from build123d import *

# Parameters (mm, degrees)
BOSS_EXTRUDE3_DEPTH = 3
FILLET1_R           = 2
SKETCH12_R          = 2.1
CUT_EXTRUDE5_DEPTH  = 10
FILLET5_R           = 4
FILLET6_R           = 3
FILLET7_R           = 10
CUT_EXTRUDE9_DEPTH  = 1.5
SKETCH17_W          = 7.951649766
SKETCH17_H          = 5.272619773
SKETCH17_W_2        = 3.894064167
SKETCH17_H_2        = 6.195846789
CUT_EXTRUDE10_DEPTH = 1.5
SKETCH18_R          = 1.6
CUT_EXTRUDE11_DEPTH = 10


with BuildPart() as part:
    # Sketch8 → Boss-Extrude3 (new body)
    with BuildSketch(Plane.XY):
        with BuildLine():
            Line((-4.848101441, -13.321505966), (-4.848101441, -0.321505966))
            add(Edge.make_bspline(
                [(-22.634292007, 16.445697007), (-22.442914483, 9.994307564), (-20.126223523, 0.876298034), (-11.53370308, 0.191019868), (-4.848101441, -0.321505966)],
                knots=[0, 0, 0, 0, 0.444535858, 1, 1, 1, 1], degree=3))
            Line((-22.634292007, 16.445697007), (-54.848101441, 16.445697007))
            Line((-54.848101441, 16.445697007), (-54.848101441, -65.321505966))
            Line((-54.848101441, -65.321505966), (-39.848101441, -65.321505966))
            Line((-39.848101441, -65.321505966), (-39.848101441, -13.321505966))
            Line((-39.848101441, -13.321505966), (-4.848101441, -13.321505966))
        make_face()
    extrude(amount=-BOSS_EXTRUDE3_DEPTH)

    # Fillet1
    fillet1_edges = [part.edges().sort_by_distance(p)[0] for p in [
        (-4.848101441, -13.321505966, -1.5),
        (-39.848101441, -65.321505966, -1.5),
        (-54.848101441, -65.321505966, -1.5),
    ]]
    fillet(fillet1_edges, radius=FILLET1_R)

    # Sketch12 → Cut-Extrude5 (cut)
    with BuildSketch(Plane.XY):
        with Locations((-47.348101441, -43.321505966)):
            Circle(SKETCH12_R)
        with Locations((-47.348101441, -59.321505966)):
            Circle(SKETCH12_R)
    extrude(amount=-CUT_EXTRUDE5_DEPTH, mode=Mode.SUBTRACT)

    # Fillet5
    fillet5_edges = [part.edges().sort_by_distance(p)[0] for p in [
        (-54.848101441, 16.445697007, -1.5),
    ]]
    fillet(fillet5_edges, radius=FILLET5_R)

    # Fillet6
    fillet6_edges = [part.edges().sort_by_distance(p)[0] for p in [
        (-4.848101441, -0.321505966, -1.5),
    ]]
    fillet(fillet6_edges, radius=FILLET6_R)

    # Fillet7
    fillet7_edges = [part.edges().sort_by_distance(p)[0] for p in [
        (-39.848101441, -13.321505966, -1.5),
    ]]
    fillet(fillet7_edges, radius=FILLET7_R)

    # Sketch16 → Cut-Extrude9 (cut)
    with BuildSketch(Plane.XY):
        with BuildLine():
            Line((-9.100213088, 21.316177145), (-9.209573917, 22.566177145))
            Line((-9.209573917, 22.566177145), (-11.640691005, 22.566177145))
            add(Edge.make_bspline(
                [(-11.640691005, 22.566177145), (-15.022495372, 19.340372794), (-15.924452017, 14.756685891)],
                knots=[0, 0, 0, 1, 1, 1], degree=2))
            ThreePointArc((-15.924452017, 14.756685891), (-15.222749011, 12.914891859), (-16.441177254, 11.365690457))
            add(Edge.make_bspline(
                [(-14.837210154, 6.041686336), (-16.459215455, 8.47618894), (-16.441177254, 11.365690457)],
                knots=[0, 0, 0, 1, 1, 1], degree=2))
            ThreePointArc((-14.837210154, 6.041686336), (-13.061711204, 6.261247316), (-11.820884577, 4.972467727))
            Line((-11.820884577, 4.972467727), (-6.820884577, 4.972467727))
            Line((-6.820884577, 4.972467727), (-6.820884577, 0.680172774))
            ThreePointArc((-6.820884577, 0.680172774), (-6.595588162, -0.64331234), (-5.945078154, -1.817709228))
            ThreePointArc((-5.945078154, -1.817709228), (-8.795904792, -7.747026555), (-11.646731431, -1.817709228))
            ThreePointArc((-11.646731431, -1.817709228), (-10.996221423, -0.64331234), (-10.770925007, 0.680172774))
            Line((-10.770925007, 0.680172774), (-10.770925007, 2.723195944))
            Line((-10.770925007, 2.723195944), (-12.604024539, 2.723195944))
            ThreePointArc((-12.604024539, 2.723195944), (-13.729925577, 2.376177145), (-14.855826616, 2.723195944))
            Line((-14.855826616, 2.723195944), (-16.623775808, 2.723195944))
            ThreePointArc((-16.623775808, 2.723195944), (-18.123775808, 2.321272155), (-19.22185202, 1.223195944))
            Line((-19.22185202, 1.223195944), (-19.272943939, 1.134702143))
            ThreePointArc((-19.272943939, 1.134702143), (-19.750526635, -0.18476513), (-19.743016315, -1.587983826))
            ThreePointArc((-19.743016315, -1.587983826), (-25.157950081, -5.408427498), (-24.556815691, 1.19126454))
            ThreePointArc((-24.556815691, 1.19126454), (-23.337837493, 1.88636976), (-22.433936663, 2.959702143))
            Line((-22.433936663, 2.959702143), (-19.683732235, 7.723195944))
            add(Edge.make_bspline(
                [(-19.683732235, 7.723195944), (-19.261177539, 8.547983183), (-18.924513654, 9.521118545), (-19.229981569, 11.075334784), (-20.358554935, 11.423731791), (-20.93203262, 11.430328812)],
                knots=[0, 0, 0, 0, 0.295584427, 0.638506801, 1, 1, 1, 1], degree=3))
            Line((-20.93203262, 11.430328812), (-22.12642518, 11.430328812))
            ThreePointArc((-22.12642518, 11.430328812), (-23.507908706, 11.184193923), (-24.719376585, 10.476080446))
            ThreePointArc((-24.719376585, 10.476080446), (-30.735444741, 13.255328812), (-24.719376585, 16.034577178))
            ThreePointArc((-24.719376585, 16.034577178), (-23.507908706, 15.326463702), (-22.12642518, 15.080328812))
            Line((-22.12642518, 15.080328812), (-20.976183849, 15.080328812))
            ThreePointArc((-20.976183849, 15.080328812), (-18.688287573, 15.799242006), (-17.222790707, 17.697563496))
            add(Edge.make_bspline(
                [(-11.640691005, 24.566177145), (-14.244308048, 22.933045591), (-16.184240838, 20.516614501), (-17.222790707, 17.697563496)],
                knots=[0, 0, 0, 0, 0.773209578, 0.773209578, 0.773209578, 0.773209578], degree=3))
            Line((-11.640691005, 24.566177145), (-8.140691005, 24.566177145))
            Line((-8.140691005, 24.566177145), (-8.140691005, 22.568020283))
            Line((-8.140691005, 22.568020283), (-8.250213088, 21.316177145))
            Line((-8.250213088, 21.316177145), (-9.100213088, 21.316177145))
        make_face()
    extrude(amount=-CUT_EXTRUDE9_DEPTH, mode=Mode.SUBTRACT)

    # Sketch17 → Cut-Extrude10 (cut)
    with BuildSketch(Plane.XY):
        with Locations((-25.46861182, 15.757865506)):
            Rectangle(SKETCH17_W, SKETCH17_H)
        with Locations((-5.398647621, -2.193777117)):
            Rectangle(SKETCH17_W_2, SKETCH17_H_2)
    extrude(amount=-CUT_EXTRUDE10_DEPTH, mode=Mode.SUBTRACT)

    # Sketch18 → Cut-Extrude11 (cut)
    with BuildSketch(Plane.XY.offset(-1.5)):
        with Locations((-27.085444741, 13.255328812)):
            Circle(SKETCH18_R)
        with Locations((-23.332950081, -2.247434774)):
            Circle(SKETCH18_R)
        with Locations((-8.795904792, -4.097026555)):
            Circle(SKETCH18_R)
    extrude(amount=-CUT_EXTRUDE11_DEPTH, mode=Mode.SUBTRACT)


solid = part.part
The listing builds one solid part. Answer for the finished solid, in the listing's coordinates (mm). A direction names the side the tool comes from. Coordinates: 2 decimals unless noted, no trailing zeros. Loops run counter-clockwise (first coordinate to the right, second up) from the corner with the lowest first, then second, coordinate; pieces in that order, holes last. Notation, with made-up numbers: (76.5, -4.5) -> (90.5, -4.5) arc R22 cw to (90.5, 18.5) -> close; hole circle Ø1 at (72, 74.5). An arc over 180 degrees is marked (long way). Write item = value, one per line. Start each with the question number.
1) A cutting plane is placed at A-A (y = -26). Give the vertices of the cut face in (x, z).
2) Given pin 1 Ø9.5 at (x, y) = (-8.8, -4.1) entering from +Z; pin 2 Ø2 at (x, y) = (-25.5, 13.5) entering from +Z; pin 3 Ø1.9 at (x, y) = (-23.33, -2.25) entering from -Z; pin 4 Ø0.5 at (x, z) = (-5, -1) entering from +Y, each flat-ended and moving along its own axis, determine where each tip first touches the part or whether it passes through.
3) A cutting plane is placed at B-B (z = -0.8). Count the separate pieces of the cut face and the enclosed holes in it, then the cut area to 3 significant figures.
4) Straight lines are drawn through the part: line 1 (X direction, y = -36, z = -0.4); line 2 (Z direction, x = -24, y = 12); line 3 (Y direction, x = -45.5, z = -1.45). For each, find the intervals that lie inside material, in ascending order. Write a range as from..to.
5) A cutting plane is placed at C-C (x = -37). Give the vertices of the cut face in (y, z), then the cut area to 3 significant figures.
6) The mould has two halves that part along Y. Classify faces 1 (the face through (-53.645, 15.305, -1.521)), 2 (the face through (-11.082, -0.866, -0.74)), 3 (the face through (-29.815, 10.832, -0.74)), 4 (the face through (-5.4, -12.7, -1.5)): released by +Y, released by -Y, zero draft, split by the parting line, or undercut.
7) A tool of negligible diameter and unlimited length cuts with its end or side. For faces 5 (the face through (-10.48, -7.335, -0.74)), 6 (the face through (-21.597, 4.41, -0.74)), 7 (the face through (-19, -13.322, -1)), from which of +Z, -Z, +X, -X, +Y, -Y can it reach the whole face along a straight path? Write none if from no direction.
Responses:
q1.outline = (-54.85, -3) -> (-39.85, -3) -> (-39.85, 0) -> (-54.85, 0) -> close
q2.pin_1 = 0
q2.pin_2 = -1.5
q2.pin_3 = through
q2.pin_4 = -5.29
q3.separate_pieces = 1
q3.enclosed_holes = 2
q3.area = 1,840 mm²
q4.line_1 = -54.85..-39.85
q4.line_2 = -3..-1.5
q4.line_3 = -65.32..-60.32, -58.32..-44.32, -42.32..16.45
q5.outline = (-16.33, -3) -> (16.45, -3) -> (16.45, 0) -> (-16.33, 0) -> close
q5.area = 98.3 mm²
q6.face_1 = released by +Y
q6.face_2 = undercut
q6.face_3 = undercut
q6.face_4 = released by -Y
q7.face_5 = +Z
q7.face_6 = +Z, +X
q7.face_7 = +Z, -Z, +X, -Y
